Read the model definition and answer for the solid it produces. Units are mm, in the model's axes. A direction names the side the tool comes from. Coordinates: 2 decimals unless noted, no trailing zeros. Write each loop counter-clockwise with the first axis right and the second up, starting at its lowest first coordinate (ties: lowest second). Pieces come first, ordered by that corner, then holes. Notation, with made-up numbers: (46, -31) -> (53, -31) arc R16 ccw to (53, -20) -> close; hole circle Ø11 at (67.25, 25). An arc over 180 degrees is marked (long way). Return JSON: item names as keys, results as strings.
from build123d import *

# Parameters (mm, degrees)
SKETCH1_W            = 100
SKETCH1_H            = 40
BOSS_EXTRUDE1_DEPTH  = 150
SKETCH2_W            = 90
SKETCH2_H            = 140
CUT_EXTRUDE1_DEPTH   = 30
SKETCH5_W            = 90
SKETCH5_H            = 10
BOSS_EXTRUDE3_DEPTH  = 30
BOSS_EXTRUDE6_DEPTH  = 6
BOSS_EXTRUDE7_DEPTH  = 3
BOSS_EXTRUDE8_DEPTH  = 6
CUT_EXTRUDE7_DEPTH   = 3
SKETCH14_W           = 3
SKETCH14_H           = 20
BOSS_EXTRUDE9_DEPTH  = 20
SKETCH15_W           = 3
SKETCH15_H           = 20
BOSS_EXTRUDE10_DEPTH = 20
SKETCH16_W           = 35
SKETCH16_H           = 2
BOSS_EXTRUDE11_DEPTH = 10
SKETCH17_W           = 35
SKETCH17_H           = 2.001720383
BOSS_EXTRUDE12_DEPTH = 10
SKETCH18_R           = 6.5
SKETCH18_R_2         = 9
CUT_EXTRUDE9_DEPTH   = 10


with BuildPart() as part:
    # Sketch1 → Boss-Extrude1 (new body)
    with BuildSketch(Plane.XY):
        with Locations((6.252485089, -6.669980119)):
            Rectangle(SKETCH1_W, SKETCH1_H)
    extrude(amount=BOSS_EXTRUDE1_DEPTH)

    # Sketch2 → Cut-Extrude1 (cut)
    with BuildSketch(Plane(origin=(0, 13.330019881, 0), x_dir=(1, 0, 0), z_dir=(0, 1, 0))):
        with Locations((6.252485089, -75)):
            Rectangle(SKETCH2_W, SKETCH2_H)
    extrude(amount=-CUT_EXTRUDE1_DEPTH, mode=Mode.SUBTRACT)

    # Sketch5 → Boss-Extrude3 (add)
    with BuildSketch(Plane(origin=(0, 13.330019881, 0), x_dir=(1, 0, 0), z_dir=(0, 1, 0))):
        with Locations((6.252485089, -110)):
            Rectangle(SKETCH5_W, SKETCH5_H)
    extrude(amount=-BOSS_EXTRUDE3_DEPTH)

    # Sketch8 → Boss-Extrude6 (add)
    with BuildSketch(Plane(origin=(0, 13.330019881, 0), x_dir=(1, 0, 0), z_dir=(0, 1, 0))):
        Polygon((-43.747514911, -113), (-43.747514911, -150), (-40.747514911, -150), (51.252485089, -150), (51.252485089, -147), (-40.747514911, -147), (-40.747514911, -113), (51.252485089, -113), (51.252485089, -110), (-43.747514911, -110), align=None)
    extrude(amount=BOSS_EXTRUDE6_DEPTH)

    # Sketch10 → Boss-Extrude7 (add)
    with BuildSketch(Plane(origin=(0, 19.330019881, 0), x_dir=(1, 0, 0), z_dir=(0, 1, 0))):
        Polygon((51.252485089, -113), (51.252485089, -115), (-38.747514911, -115), (-38.747514911, -145), (51.252485089, -145), (51.252485089, -147), (-40.747514911, -147), (-40.747514911, -113), align=None)
    extrude(amount=-BOSS_EXTRUDE7_DEPTH)

    # Sketch11 → Boss-Extrude8 (add)
    with BuildSketch(Plane(origin=(0, 19.330019881, 0), x_dir=(1, 0, 0), z_dir=(0, 1, 0))):
        Polygon((51.252485089, -110), (51.252485089, -105), (-38.747514911, -105), (-38.747514911, -5), (51.252485089, -5), (51.252485089, 0), (-43.747514911, 0), (-43.747514911, -110), align=None)
    extrude(amount=-BOSS_EXTRUDE8_DEPTH)

    # Sketch13 → Cut-Extrude7 (cut)
    with BuildSketch(Plane(origin=(0, 13.330019881, 0), x_dir=(1, 0, 0), z_dir=(0, 1, 0))):
        Polygon((51.252485089, -3), (-40.747514911, -3), (-40.747514911, -107), (51.252485089, -107), (51.252485089, -105), (-38.747514911, -105), (-38.747514911, -5), (51.252485089, -5), align=None)
    extrude(amount=CUT_EXTRUDE7_DEPTH, mode=Mode.SUBTRACT)

    # Sketch14 → Boss-Extrude9 (add)
    with BuildSketch(Plane(origin=(0, -16.669980119, 0), x_dir=(1, 0, 0), z_dir=(0, 1, 0))):
        with Locations((-32.747514911, -130)):
            Rectangle(SKETCH14_W, SKETCH14_H)
    extrude(amount=BOSS_EXTRUDE9_DEPTH)

    # Sketch15 → Boss-Extrude10 (add)
    with BuildSketch(Plane(origin=(0, -16.669980119, 0), x_dir=(1, 0, 0), z_dir=(0, 1, 0))):
        with Locations((45.252485089, -130)):
            Rectangle(SKETCH15_W, SKETCH15_H)
    extrude(amount=BOSS_EXTRUDE10_DEPTH)

    # Sketch16 → Boss-Extrude11 (add)
    with BuildSketch(Plane(origin=(0, -16.669980119, 0), x_dir=(1, 0, 0), z_dir=(0, 1, 0))):
        with Locations((6.252485089, -121)):
            Rectangle(SKETCH16_W, SKETCH16_H)
    extrude(amount=BOSS_EXTRUDE11_DEPTH)

    # Sketch17 → Boss-Extrude12 (add)
    with BuildSketch(Plane(origin=(0, -16.669980119, 0), x_dir=(1, 0, 0), z_dir=(0, 1, 0))):
        with Locations((6.252485089, -138.999139808)):
            Rectangle(SKETCH17_W, SKETCH17_H)
    extrude(amount=BOSS_EXTRUDE12_DEPTH)

    # Sketch18 → Cut-Extrude9 (cut)
    with BuildSketch(Plane.XY):
        with Locations((6.252485089, -1.669980119)):
            Circle(SKETCH18_R)
        with Locations((36.752485089, -1.669980119)):
            Circle(SKETCH18_R_2)
        with Locations((-24.247514911, -1.669980119)):
            Circle(SKETCH18_R_2)
    extrude(amount=CUT_EXTRUDE9_DEPTH, mode=Mode.SUBTRACT)


solid = part.part
1. Consider L1, parallel to Z at x = 25, y = 14.5; L2, parallel to Z at x = -15, y = -15.5; L3, parallel to X at y = 1.5, z = 122. Determine where each line is inside the solid, lowest interval first.
Taken from the geometry:
{"L1": "z = 0 to 3, 107 to 113, 147 to 150", "L2": "z = 0 to 5, 105 to 115, 145 to 150", "L3": "x = -43.75 to -38.75, -34.25 to -31.25, 43.75 to 46.75, 51.25 to 56.25"}
2. The part is cut by section C-C (x = 49.5). Determine the outline of the cut face in (y, z).
Taken from the geometry:
{"outline": "(-26.67, 0) -> (19.33, 0) -> (19.33, 5) -> (16.33, 5) -> (16.33, 3) -> (13.33, 3) -> (13.33, 5) -> (-16.67, 5) -> (-16.67, 105) -> (13.33, 105) -> (13.33, 107) -> (16.33, 107) -> (16.33, 105) -> (19.33, 105) -> (19.33, 115) -> (16.33, 115) -> (16.33, 113) -> (13.33, 113) -> (13.33, 115) -> (-16.67, 115) -> (-16.67, 145) -> (13.33, 145) -> (13.33, 147) -> (16.33, 147) -> (16.33, 145) -> (19.33, 145) -> (19.33, 150) -> (-26.67, 150) -> close"}
3. Flat-ended cylindrical pins translate along their axes: pin 1 Ø1.5 at (x, y) = (3.5, -6.5) entering from -Z; pin 2 Ø9 at (x, z) = (22.5, 131.5) entering from +Y; pin 3 Ø15 at (x, y) = (11.5, 5.5) entering from -Z; pin 4 Ø1 at (x, z) = (7.5, 121.5) entering from +Y. Find the tip coordinate at first contact, or state that the pin passes through.
Taken from the geometry:
{"pin 1": "stops at z = 105", "pin 2": "stops at y = -16.67", "pin 3": "stops at z = 0", "pin 4": "stops at y = -6.67"}
4. The part is cut by section A-A (y = -13). Determine the outline of the cut face in (x, z), then the cut area to 3 significant figures.
Taken from the geometry:
{"outline": "(-43.75, 0) -> (56.25, 0) -> (56.25, 150) -> (-43.75, 150) -> close; (-34.25, 120) -> (-31.25, 120) -> (-31.25, 140) -> (-34.25, 140) -> close; (-11.25, 120) -> (23.75, 120) -> (23.75, 122) -> (-11.25, 122) -> close; (-11.25, 138) -> (23.75, 138) -> (23.75, 140) -> (-11.25, 140) -> close; (43.75, 120) -> (46.75, 120) -> (46.75, 140) -> (43.75, 140) -> close; hole (-38.75, 5) -> (51.25, 5) -> (51.25, 105) -> (-38.75, 105) -> close; hole (-38.75, 115) -> (51.25, 115) -> (51.25, 145) -> (-38.75, 145) -> close", "area": "3,560 mm2"}
5. The part is cut by section B-B (z = 23). Determine the outline of the cut face in (x, y).
Taken from the geometry:
{"outline": "(-43.75, -26.67) -> (56.25, -26.67) -> (56.25, 13.33) -> (51.25, 13.33) -> (51.25, -16.67) -> (-38.75, -16.67) -> (-38.75, 13.33) -> (-40.75, 13.33) -> (-40.75, 16.33) -> (-38.75, 16.33) -> (-38.75, 19.33) -> (-43.75, 19.33) -> close"}
6. A tool of negligible diameter and unlimited length cuts with its end or side. For faces 1 (the face through (-40.748, 15, 130)), 2 (the face through (51.252, -1, 130)), 3 (the face through (-15.66, 1.03, 2.46)), from which of +Z, -Z, +X, -X, +Y, -Y can it reach the whole face along a straight path? Write none if from no direction.
Taken from the geometry:
{"face 1": "+X", "face 2": "+Y", "face 3": "-Z"}
7. For a pull along X with two mould halves and no side action, classify faces 4 (the face through (7, 18, 115)), 5 (the face through (6, -1, 115)), 6 (the face through (-38.748, 18, 56)) as +X half, -X half, draft (parallel to the pull), parting line (faces both ways), or undercut.
Taken from the geometry:
{"face 4": "draft", "face 5": "undercut", "face 6": "+X half"}
